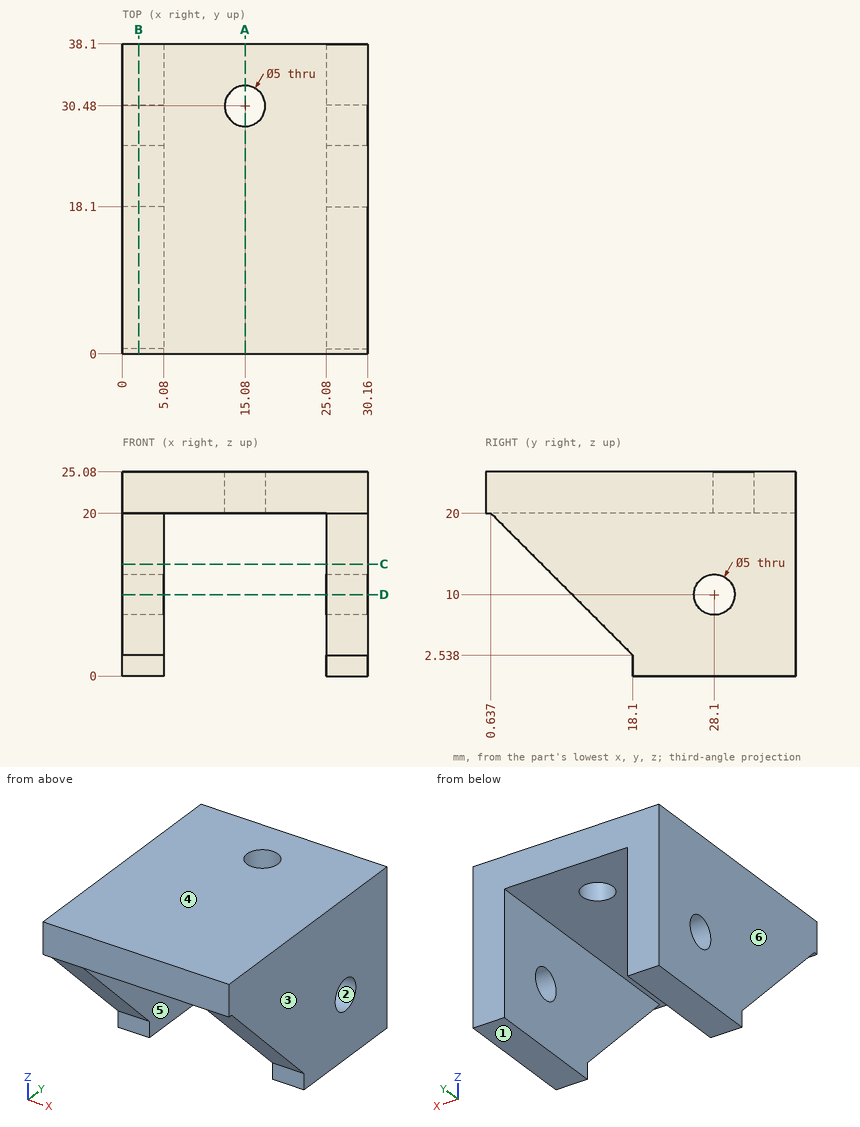
Input: dimensioned drawing with shaded views. Units: mm. Origin: part minimum x, y, z. A direction names the side the tool comes from. Give positions to 0.01 mm unless a question says otherwise; leave off trailing zeros. Write each loop counter-clockwise with the first axis right and the second up, starting at its lowest first coordinate (ties: lowest second). Pieces come first, ordered by that corner, then holes. Notation, with made-up numbers: (42.25, 84.25) - (87.25, 84.25) arc R12 cw to (87.25, 96.25) - close; hole circle Ø5 at (-35, 24). An arc over 180 degrees is marked (long way). One line per item, written item: value. Start each with the question number.
Q1. Section query B-B, the plane x = 2. Return the cut outline in (y, z).
Q2. Section query A-A, the plane x = 15.08. Return the cut outline in (y, z).
Q3. Draft query along Z for the marked faces 1, 2, 3 and 4. Return one class per face: +Z half, -Z half, draft (parallel to the pull), parting line (faces both ways), or undercut.
Q4. Section query C-C, the plane z = 13.75. Return the cut outline in (x, y), then the cut area to 3 significant figures.
Q5. First-contact query: pin 1 Ø1.3 at (x, z) = (28.5, 1.5) entering from -Y; pin 2 Ø2 at (x, y) = (11.5, 24.5) entering from -Z; pin 3 Ø3 at (y, z) = (28.1, 10) entering from +X. Flat tips, straight axial feed; report the tip coordinate or a pass-through.
Q6. Section query D-D, the plane z = 10. Return the cut outline in (x, y), then the cut area to 3 significant figures.
Q7. Set-up query: the marked faces 5 and 6. Return all of +Z, -Z, +X, -X, +Y, -Y with unobstructed straight access to the full face (end or side cutting, diameter ignored); none if empty.
Q8. Material intervals for probe 1 along Y at (x, z) = (15.08, 22.1); probe 2 along X at (y, z) = (30.48, 23.55); probe 3 along X at (y, z) = (10.5, 19.75), sorted ascending. Write a range as from..to.
Answer:
1. outline: (0, 20) - (0.64, 20) - (18.1, 2.54) - (18.1, 0) - (38.1, 0) - (38.1, 25.08) - (0, 25.08) - close; hole circle Ø5 at (28.1, 10)
2. outline: (0, 20) - (27.98, 20) - (27.98, 25.08) - (0, 25.08) - close; (32.98, 20) - (38.1, 20) - (38.1, 25.08) - (32.98, 25.08) - close
3. face 1: -Z half
3. face 2: undercut
3. face 3: draft
3. face 4: +Z half
4. outline: (0, 6.89) - (5.08, 6.89) - (5.08, 38.1) - (0, 38.1) - close; (25.08, 6.89) - (30.16, 6.89) - (30.16, 38.1) - (25.08, 38.1) - close
4. area: 317 mm2
5. pin 1: stops at y = 18.1
5. pin 2: stops at z = 20
5. pin 3: passes through
6. outline: (0, 10.64) - (5.08, 10.64) - (5.08, 25.6) - (0, 25.6) - close; (0, 30.6) - (5.08, 30.6) - (5.08, 38.1) - (0, 38.1) - close; (25.08, 10.64) - (30.16, 10.64) - (30.16, 25.6) - (25.08, 25.6) - close; (25.08, 30.6) - (30.16, 30.6) - (30.16, 38.1) - (25.08, 38.1) - close
6. area: 228 mm2
7. face 5: -Z, +Y, -Y
7. face 6: +Z, -Z, -X, +Y, -Y
8. probe 1: y = 0..27.98, 32.98..38.1
8. probe 2: x = 0..12.58, 17.58..30.16
8. probe 3: x = 0..5.08, 25.08..30.16
